from build123d import *

# Parameters (mm, degrees)
SKETCH1_W             = 60.9
SKETCH1_H             = 25.2
BOSS_EXTRUDE1_DEPTH   = 4
SKETCH3_R             = 4
SKETCH3_R_2           = 2.15
CUT_EXTRUDE1_DEPTH    = 2.6
SKETCH3_2_R           = 2.15
CUT_EXTRUDE2_DEPTH    = 67.029160225
SKETCH4_W             = 19.2
SKETCH4_H             = 7.5
BOSS_EXTRUDE2_DEPTH   = 60.9
SKETCH5_R             = 4.9
CUT_EXTRUDE3_DEPTH    = 2
M5X0_8_TAPPED_HOLE1_D = 4.2
FILLET1_R             = 2
FILLET2_R             = 3.6


with BuildPart() as part:
    # Sketch1 → Boss-Extrude1 (new body)
    with BuildSketch(Plane.XY):
        with Locations((30.45, -12.6)):
            Rectangle(SKETCH1_W, SKETCH1_H)
    extrude(amount=-BOSS_EXTRUDE1_DEPTH)

    # Sketch3 → Cut-Extrude1 (cut)
    # profile 1 of 3: a face of its own
    with BuildSketch(Plane.XY):
        with Locations((9.2, -18)):
            Circle(SKETCH3_R)
        with Locations((9.2, -18)):
            Circle(SKETCH3_R_2, mode=Mode.SUBTRACT)
    # profile 2 of 3: a face of its own
    with BuildSketch(Plane.XY):
        with Locations((29.1, -18)):
            Circle(SKETCH3_R)
        with Locations((29.1, -18)):
            Circle(SKETCH3_R_2, mode=Mode.SUBTRACT)
    # profile 3 of 3: a face of its own
    with BuildSketch(Plane.XY):
        with Locations((49, -18)):
            Circle(SKETCH3_R)
        with Locations((49, -18)):
            Circle(SKETCH3_R_2, mode=Mode.SUBTRACT)
    extrude(amount=-CUT_EXTRUDE1_DEPTH, mode=Mode.SUBTRACT)

    # Sketch3<2> → Cut-Extrude2 (cut, through all)
    with BuildSketch(Plane.XY):
        with Locations((9.2, -18)):
            Circle(SKETCH3_2_R)
        with Locations((29.1, -18)):
            Circle(SKETCH3_2_R)
        with Locations((49, -18)):
            Circle(SKETCH3_2_R)
    extrude(amount=-CUT_EXTRUDE2_DEPTH, mode=Mode.SUBTRACT)

    # Sketch4 → Boss-Extrude2 (add)
    with BuildSketch(Plane.ZY):
        with Locations((-13.6, -3.75)):
            Rectangle(SKETCH4_W, SKETCH4_H)
    extrude(amount=-BOSS_EXTRUDE2_DEPTH)

    # Sketch5 → Cut-Extrude3 (cut)
    with BuildSketch(Plane(origin=(0, 0, 0), x_dir=(1, 0, 0), z_dir=(0, 1, 0))):
        with Locations(Location((10.16, 17.42, 0), (0, 0, 270))):
            Circle(SKETCH5_R)
        with Locations(Location((50.8, 17.42, 0), (0, 0, 270))):
            Circle(SKETCH5_R)
    extrude(amount=-CUT_EXTRUDE3_DEPTH, mode=Mode.SUBTRACT)

    # M5x0.8 Tapped Hole1 (through all)
    with Locations(Plane(origin=(0, -2, 0), x_dir=(1, 0, 0), z_dir=(0, 1, 0))):
        with Locations((10.16, 17.42), (50.8, 17.42)):
            Hole(M5X0_8_TAPPED_HOLE1_D / 2)

    # Fillet1
    # the kernel refuses this fillet: 2 mm, written as the material it takes off along each edge
    with BuildSketch(Plane(origin=(-5, 0, -23.2), x_dir=(0, 0, 1), z_dir=(1, 0, 0)), Plane(origin=(-5, -7.5, -23.2), x_dir=(0, 1, 0), z_dir=(1, 0, 0)), Plane(origin=(65.9, -25.2, -4), x_dir=(0, 0, 1), z_dir=(-1, 0, 0))) as fillet1_piece_1:
        with BuildLine():
            CenterArc((FILLET1_R, FILLET1_R), FILLET1_R, 180, 90)
            Line((0, FILLET1_R), (0, 0))
            Line((0, 0), (FILLET1_R, 0))
        make_face()
    extrude(amount=70.9, mode=Mode.SUBTRACT)

    # Fillet2
    fillet2_edges = [part.edges().sort_by_distance(p)[0] for p in [
        (30.45, -7.5, -4),
    ]]
    fillet(fillet2_edges, radius=FILLET2_R)


solid = part.part
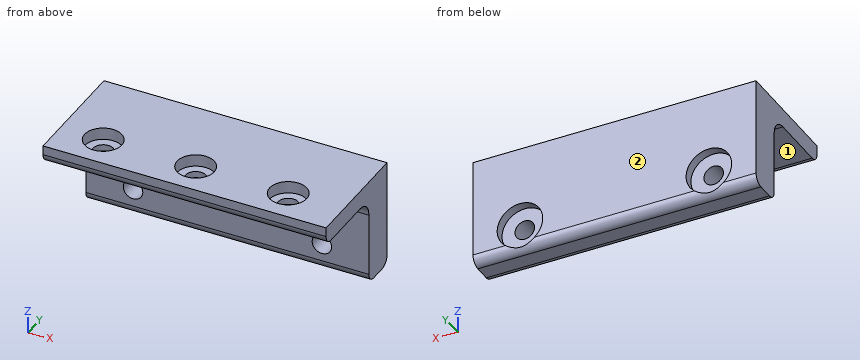
Model file for the job. Use its own axes, mm. Face numbers are marked on the shaded views. A direction names the side the tool comes from. Round coordinates to 2 decimals unless told otherwise and drop trailing zeros. Loops run counter-clockwise (first coordinate to the right, second up) from the corner with the lowest first, then second, coordinate; pieces in that order, holes last.
1. Band-saw the part on D-D, the plane y = -2.75. List the corners of the cut face in (x, z).
Check values:
outline: (0, -23.2) - (60.9, -23.2) - (60.9, 0) - (0, 0) - close; hole circle Ø4.2 at (10.16, -17.42); hole circle Ø4.2 at (50.8, -17.42)
2. Band-saw the part on B-B, the plane x = 49.5. List the corners of the cut face in (y, z).
Check values:
outline: (-25.2, -2) arc R2 ccw to (-23.2, -4) - (-20.09, -4) - (-20.09, -2.6) - (-21.97, -2.6) - (-21.97, 0) - (-25.2, 0) - close; (-15.91, -4) - (-11.1, -4) arc R3.6 cw to (-7.5, -7.6) - (-7.5, -15.77) - (-2, -15.77) - (-2, -12.7) - (0, -12.7) - (0, 0) - (-14.03, 0) - (-14.03, -2.6) - (-15.91, -2.6) - close; (-7.5, -21.2) arc R2 ccw to (-5.5, -23.2) - (-2, -23.2) arc R2 ccw to (-0.24, -22.14) - (-2, -22.14) - (-2, -19.07) - (-7.5, -19.07) - close
3. Band-saw the part on C-C, the plane y = -18. List the corners of the cut face in (x, z), and give its area (3 significant figures).
Check values:
outline: (0, -4) - (7.05, -4) - (7.05, -2.6) - (5.2, -2.6) - (5.2, 0) - (0, 0) - close; (11.35, -4) - (26.95, -4) - (26.95, -2.6) - (25.1, -2.6) - (25.1, 0) - (13.2, 0) - (13.2, -2.6) - (11.35, -2.6) - close; (31.25, -4) - (46.85, -4) - (46.85, -2.6) - (45, -2.6) - (45, 0) - (33.1, 0) - (33.1, -2.6) - (31.25, -2.6) - close; (51.15, -4) - (60.9, -4) - (60.9, 0) - (53, 0) - (53, -2.6) - (51.15, -2.6) - close
area: 163 mm2
4. Tool access for the marked faces 1 and 2: list every direction of +Z, -Z, +X, -X, +Y, -Y with a clear straight run to the whole face (end or side of a thin tool).
Check values:
face 1: -Z, +X, -X, -Y
face 2: +Z, -Z, +X, -X, +Y
5. Drop flat-ended pins along their axis: P1, Ø5.5, axis at x = 10.16, z = -17.42, coming from the -Y side; P2, Ø5, axis at x = 9.2, y = -18, coming from the -Z side; P3, Ø2.5, axis at x = 50.5, y = -16.5, coming from the +Z side. Give the stop position or say it passes through.
Check values:
P1: stops at y = -7.5
P2: stops at z = -4
P3: stops at z = -2.6
6. Band-saw the part on A-A, the plane z = -17.42. List the corners of the cut face in (x, y), and give its area (3 significant figures).
Check values:
outline: (0, -7.5) - (8.06, -7.5) - (8.06, -2) - (5.26, -2) - (5.26, 0) - (0, 0) - close; (12.26, -7.5) - (48.7, -7.5) - (48.7, -2) - (45.9, -2) - (45.9, 0) - (15.06, 0) - (15.06, -2) - (12.26, -2) - close; (52.9, -7.5) - (60.9, -7.5) - (60.9, 0) - (55.7, 0) - (55.7, -2) - (52.9, -2) - close
area: 371 mm2
7. Wall check: probe 1 along X at (y, z) = (-1.5, -17.42); probe 2 along Y at (x, z) = (9.2, -0.6); probe 3 along Y at (x, z) = (16, -18.5). Give the ranges that are in metal, low to high.
Check values:
probe 1: x = 0 to 5.26, 15.06 to 45.9, 55.7 to 60.9
probe 2: y = -25.2 to -22, -14 to 0
probe 3: y = -7.5 to 0
